Design review of the part built by this model. Coordinates are the model's own, in mm. Face numbers are marked on the shaded views. A direction names the side the tool comes from. Round coordinates to 2 decimals unless told otherwise and drop trailing zeros. Write each loop counter-clockwise with the first axis right and the second up, starting at its lowest first coordinate (ties: lowest second). Pieces come first, ordered by that corner, then holes. Notation, with made-up numbers: (-17.5, 13.5) -> (38.5, 13.5) arc R27 ccw to (38.5, 35.5) -> close; hole circle Ø5 at (43, 44). An arc over 180 degrees is marked (long way). One line per question, with ' | ' between items. Start each with the question number.
1) Consider section A-A (x = 5.75). Give the boundary of the cut face in (y, z).
2) For probe 1 along Y at (x, z) = (5.75, 1.25); probe 2 along X at (y, z) = (23.5, 2.4); probe 3 along X at (y, z) = (10, 1.3), list the stretches that pass through material, from the lowest coordinate up.
3) Consider section C-C (y = 4.5). Give the boundary of the cut face in (x, z).
4) Consider section D-D (y = 14). Give the boundary of the cut face in (x, z).
5) For the marked faces 4, 5, 6, 7 and 8, list the 3-axis set-ups (+Z, -Z, +X, -X, +Y, -Y) from which the entire face can be reached by the end or side of a thin tool; tool diameter is ignored.
6) Consider section B-B (z = 1.6). Give the boundary of the cut face in (x, y).
7) Mouldability with a two-part tool opening along X and no side actions: class the marked faces 1, 2 and 3 as +X half, -X half, draft (parallel to the pull), parting line (faces both ways), or undercut.
8) Insertion check: pin 1 Ø0.6 at (x, z) = (12, 1.5) entering from -Y; pin 2 Ø1.5 at (y, z) = (17, 2) entering from -X; pin 3 Ø0.6 at (y, z) = (23, 1.5) entering from +X; pin 4 Ø3.5 at (x, y) = (5.75, 4.5) entering from -Z. Each pin has a flat end and moves straight along its axis. Give the tip position at first contact, or say it passes through.
```python
from build123d import *

# Parameters (mm, degrees)
ESBO_O1_R                = 1.5
RESSALTO_EXTRUS_O1_DEPTH = 3
FILETE1_R                = 2
FILETE2_R                = 2


with BuildPart() as part:
    # Esboço1 → Ressalto-extrusão1 (new body)
    with BuildSketch(Plane.XY):
        Polygon((11.5, 28), (13.55, 28), (13.55, 31.5), (-2.05, 31.5), (-2.05, 28), (0, 28), (0, 0), (11.5, 0), align=None)
        with Locations((5.75, 4.5)):
            Circle(ESBO_O1_R, mode=Mode.SUBTRACT)
        with BuildLine():
            Line((4.25, 21.5), (4.25, 23.5))
            ThreePointArc((4.25, 23.5), (5.75, 25), (7.25, 23.5))
            Line((7.25, 23.5), (7.25, 21.5))
            ThreePointArc((7.25, 21.5), (5.75, 20), (4.25, 21.5))
        make_face(mode=Mode.SUBTRACT)
    extrude(amount=RESSALTO_EXTRUS_O1_DEPTH)

    # Filete1
    filete1_edges = [part.edges().sort_by_distance(p)[0] for p in [
        (-2.05, 31.5, 1.5),
        (13.55, 31.5, 1.5),
    ]]
    fillet(filete1_edges, radius=FILETE1_R)

    # Filete2
    filete2_edges = [part.edges().sort_by_distance(p)[0] for p in [
        (11.5, 0, 1.5),
        (0, 0, 1.5),
    ]]
    fillet(filete2_edges, radius=FILETE2_R)


solid = part.part
```
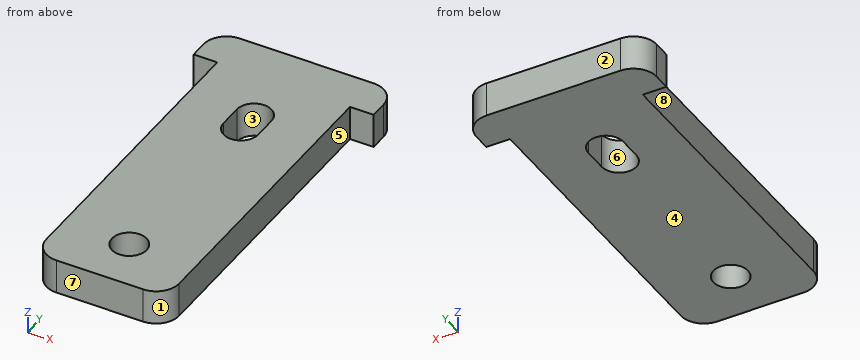
From the geometry:
1) outline: (0, 0) -> (3, 0) -> (3, 3) -> (0, 3) -> close; (6, 0) -> (20, 0) -> (20, 3) -> (6, 3) -> close; (25, 0) -> (31.5, 0) -> (31.5, 3) -> (25, 3) -> close
2) probe 1: y = 0 to 3, 6 to 20, 25 to 31.5 | probe 2: x = 0 to 4.25, 7.25 to 11.5 | probe 3: x = 0 to 11.5
3) outline: (0, 0) -> (4.25, 0) -> (4.25, 3) -> (0, 3) -> close; (7.25, 0) -> (11.5, 0) -> (11.5, 3) -> (7.25, 3) -> close
4) outline: (0, 0) -> (11.5, 0) -> (11.5, 3) -> (0, 3) -> close
5) face 4: -Z, +X, -X, +Y, -Y | face 5: +Z, -Z, +X, -Y | face 6: +Z, -Z | face 7: +Z, -Z, +X, -X, -Y | face 8: +Z, -Z, -X, -Y
6) outline: (-2.05, 28) -> (0, 28) -> (0, 2) arc R2 ccw to (2, 0) -> (9.5, 0) arc R2 ccw to (11.5, 2) -> (11.5, 28) -> (13.55, 28) -> (13.55, 29.5) arc R2 ccw to (11.55, 31.5) -> (-0.05, 31.5) arc R2 ccw to (-2.05, 29.5) -> close; hole circle Ø3 at (5.75, 4.5); hole (4.25, 21.5) arc R1.5 ccw to (7.25, 21.5) -> (7.25, 23.5) arc R1.5 ccw to (4.25, 23.5) -> close
7) face 1: +X half | face 2: draft | face 3: undercut
8) pin 1: stops at y = 28 | pin 2: stops at x = 0 | pin 3: stops at x = 11.5 | pin 4: stops at z = 0
